from build123d import *

# Parameters (mm, degrees)
F0_R     = 15.875
F1_DEPTH = 1828.8
F4_R     = 15.875
F6_COUNT = 3


with BuildPart() as f1:
    # F0 (on Top) → F1 (new body)
    with BuildSketch(Plane.XY):
        Circle(F0_R)
    extrude(amount=F1_DEPTH)

    # F5: sweep along a path in F2
    with BuildLine(Plane.XZ) as f5_path:
        Line((0, 609.6), (457.2, 0))
    # F4 (on face) → F5 (sweep)
    with BuildSketch(Plane(origin=(164.592, 0, -219.456), x_dir=(0.8, 0, 0.6), z_dir=(0.6, 0, -0.8))):
        with Locations((365.76, 0)):
            Circle(F4_R)
    sweep(path=f5_path.line)

    # F6: F1 ×3 about axis
    f6_axis = Axis((0, 0, 0), (0, 0, -1))


with BuildPart() as f1_1:
    add(f1.part)
    for i in range(1, F6_COUNT):
        add(f1.part.rotate(f6_axis, i * 360 / F6_COUNT))


solid = f1_1.part
Build history of the part. All positions in model axes, mm. Give positions to 0.01 mm unless a question says otherwise; leave off trailing zeros. Order: outer loops, then holes, each group sorted by start corner. A loop starts at its lowest first (then second) coordinate and runs counter-clockwise, first axis right, second up. Notation, with made-up numbers: M 57.25,56 L 95.25,56 A28 ccw 95.25,93 Z; hole C 7,22.5 d3. An arc over 180 degrees is marked long. Put each result on its own line as item: value.
Item 1: Probe line 1 (Z direction, x = 387.5, y = -6). List the from-to ranges inside material, lowest first. Write a range as [from, to].
From the geometry:
line 1: z = [68.44, 117.43]
Item 2: Slice it at B-B, the plane z = 363. Give the number of separate pieces and of enclosed holes in the cut face, plus the area to 3 significant figures.
From the geometry:
separate pieces: 4
enclosed holes: 0
area: 3,760 mm2
Item 3: Slice it at A-A, the plane z = 1475.5. Write the cut outline in (x, y) (3 decimals).
From the geometry:
outline: C 0,0 d31.75
